```python
from build123d import *

# Parameters (mm, degrees)
STOCK_DGT_START                               = 10.16
STOCK_DGT_INSIDE_SWERVE_STRUCTURE_SM_2_R      = 1.905
STOCK_DGT_INSIDE_SWERVE_STRUCTURE_SM_2_R_2    = 1.5
STOCK_DGT_INSIDE_SWERVE_STRUCTURE_SM_2_R_3    = 4.7625
STOCK_DGT_INSIDE_SWERVE_STRUCTURE_SMALL_DEPTH = 2.286
CUT_EXTRUDE2_DEPTH                            = 66.309248357
FILLET1_R                                     = 2.54
FILLET2_R                                     = 1.27
CHAMFER1_SIZE                                 = 1.27


# Read off the part's stored shape, not the designer's step: Stock-DGT inside swerve structure Small Bearing-1
with BuildPart() as part:
    # Stock-DGT inside swerve structure Sm 2 → Stock-DGT inside swerve structure Small Bearing-1 (new body)
    with BuildSketch(Plane.YZ.offset(STOCK_DGT_START)):
        with BuildLine():
            ThreePointArc((34.33064, -8.13506567), (36.425690436, -10.904598407), (39.07282, -13.152320138))
            Line((39.07282, -13.152320138), (39.07282, -21.59))
            Line((39.07282, -21.59), (56.85282, -21.59))
            Line((56.85282, -21.59), (56.85282, -13.152320138))
            ThreePointArc((56.85282, -13.152320138), (59.499949564, -10.904598407), (61.595, -8.13506567))
            Line((61.595, -8.13506567), (61.595, 8.13506567))
            ThreePointArc((61.595, 8.13506567), (59.499949564, 10.904598407), (56.85282, 13.152320138))
            Line((56.85282, 13.152320138), (56.85282, 21.59))
            Line((56.85282, 21.59), (39.07282, 21.59))
            Line((39.07282, 21.59), (39.07282, 13.152320138))
            ThreePointArc((39.07282, 13.152320138), (36.425690436, 10.904598407), (34.33064, 8.13506567))
            Line((34.33064, 8.13506567), (34.33064, -8.13506567))
        make_face()
        with Locations((42.56532, -18.288)):
            Circle(STOCK_DGT_INSIDE_SWERVE_STRUCTURE_SM_2_R, mode=Mode.SUBTRACT)
        with Locations((41.245305579, -6.717514421)):
            Circle(STOCK_DGT_INSIDE_SWERVE_STRUCTURE_SM_2_R_2, mode=Mode.SUBTRACT)
        with Locations((53.36032, -18.288)):
            Circle(STOCK_DGT_INSIDE_SWERVE_STRUCTURE_SM_2_R, mode=Mode.SUBTRACT)
        with Locations((53.619674249, -5.656854249)):
            Circle(STOCK_DGT_INSIDE_SWERVE_STRUCTURE_SM_2_R_2, mode=Mode.SUBTRACT)
        with Locations((42.305965751, 5.656854249)):
            Circle(STOCK_DGT_INSIDE_SWERVE_STRUCTURE_SM_2_R_2, mode=Mode.SUBTRACT)
        with Locations((42.56532, 18.288)):
            Circle(STOCK_DGT_INSIDE_SWERVE_STRUCTURE_SM_2_R, mode=Mode.SUBTRACT)
        with Locations((47.96282, 0)):
            Circle(STOCK_DGT_INSIDE_SWERVE_STRUCTURE_SM_2_R_3, mode=Mode.SUBTRACT)
        with Locations((54.680334421, 6.717514421)):
            Circle(STOCK_DGT_INSIDE_SWERVE_STRUCTURE_SM_2_R_2, mode=Mode.SUBTRACT)
        with Locations((53.36032, 18.288)):
            Circle(STOCK_DGT_INSIDE_SWERVE_STRUCTURE_SM_2_R, mode=Mode.SUBTRACT)
    extrude(amount=STOCK_DGT_INSIDE_SWERVE_STRUCTURE_SMALL_DEPTH)

    # Sketch2 → Cut-Extrude2 (cut, through all)
    with BuildSketch(Plane.ZY.offset(-10.16)):
        with BuildLine():
            Line((-12.844591897, 56.85282), (-13.152320138, 56.85282))
            ThreePointArc((-13.152320138, 56.85282), (0, 63.83782), (13.152320138, 56.85282))
            Line((13.152320138, 56.85282), (12.844591897, 56.85282))
            ThreePointArc((12.844591897, 56.85282), (0, 63.58382), (-12.844591897, 56.85282))
        make_face()
        with BuildLine():
            Line((13.152320138, 39.07282), (12.844591897, 39.07282))
            ThreePointArc((12.844591897, 39.07282), (0, 32.34182), (-12.844591897, 39.07282))
            Line((-12.844591897, 39.07282), (-13.152320138, 39.07282))
            ThreePointArc((-13.152320138, 39.07282), (0, 32.08782), (13.152320138, 39.07282))
        make_face()
    extrude(amount=-CUT_EXTRUDE2_DEPTH, mode=Mode.SUBTRACT)

    # Fillet1
    fillet1_edges = [part.edges().sort_by_distance(p)[0] for p in [
        (11.303, 34.33064, 7.627536263),
        (11.303, 34.33064, -7.627536263),
        (11.303, 61.595, -7.627536263),
        (11.303, 61.595, 7.627536263),
        (11.303, 56.85282, 12.844591897),
        (11.303, 56.85282, -12.844591897),
        (11.303, 39.07282, -12.844591897),
        (11.303, 39.07282, 12.844591897),
    ]]
    fillet(fillet1_edges, radius=FILLET1_R)

    # Fillet2
    fillet2_edges = [part.edges().sort_by_distance(p)[0] for p in [
        (11.303, 39.07282, 21.59),
        (11.303, 56.85282, 21.59),
        (11.303, 56.85282, -21.59),
        (11.303, 39.07282, -21.59),
    ]]
    fillet(fillet2_edges, radius=FILLET2_R)

    # Chamfer1
    chamfer1_edges = [part.edges().sort_by_distance(p)[0] for p in [
        (12.446, 51.45532, 18.288),
        (12.446, 40.66032, -18.288),
        (12.446, 51.45532, -18.288),
        (12.446, 40.66032, 18.288),
    ]]
    chamfer(chamfer1_edges, length=CHAMFER1_SIZE)


solid = part.part
```
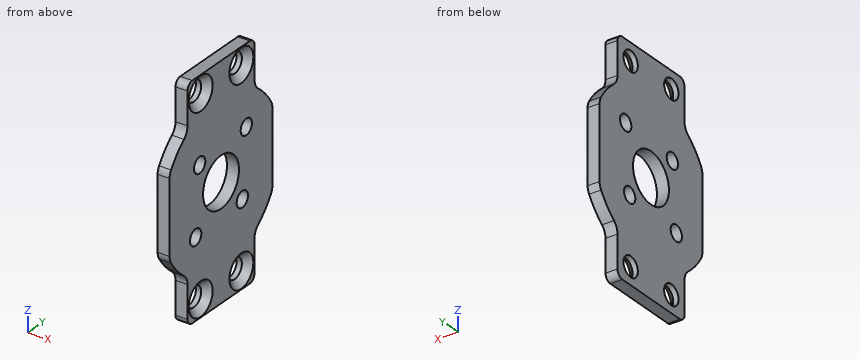
CAD build for the part. Positions are in the model's coordinates, mm. Round coordinates to 2 decimals unless told otherwise and drop trailing zeros. Order: outer loops, then holes, each group sorted by start corner. A loop starts at its lowest first (then second) coordinate and runs counter-clockwise, first axis right, second up.
Item 1: Saw through at B-B on x = 10.65. State how many separate pieces and enclosed holes the cut face has, then the cut area to 3 significant figures.
Item 2: Saw through at A-A on z = 0. Write the cut outline in (x, y) (3 decimals), then the cut area to 3 significant figures.
Item 3: Probe line 1 along Z through (x, y) = (11.75, 55.5); line 2 along Y through (x, z) = (11.9, -6) (3 decimals); line 3 along Y through (x, z) = (11.45, -15.5). List the from-to ranges inside material, lowest first.
Item 4: Pin check, flat tips, straight feed: pin 1 (1.8 mm diameter, centred on y = 53.62, z = -5.66, fed in from -X); pin 2 (1.1 mm diameter, centred on x = 11, z = 17.5, fed in from -Y); pin 3 (6 mm diameter, centred on y = 53.36, z = -18.29, fed in from +X); pin 4 (1.1 mm diameter, centred on x = 11, z = 16.5, fed in from +Y). Stop position of each tip, or through.
Reported:
1. separate pieces: 1
1. enclosed holes: 9
1. area: 824 mm2
2. outline: (10.16, 34.331) - (12.446, 34.331) - (12.446, 43.2) - (10.16, 43.2) - close; (10.16, 52.725) - (12.446, 52.725) - (12.446, 61.595) - (10.16, 61.595) - close
2. area: 40.6 mm2
3. line 1: z = -21.59 to -19.54, -17.04 to 5.46, 7.97 to 17.04, 19.54 to 21.59
3. line 2: y = 34.331 to 39.928, 42.563 to 52.159, 55.08 to 61.595
3. line 3: y = 39.07 to 56.85
4. pin 1: passes through
4. pin 2: stops at y = 39.07
4. pin 3: stops at x = 12.27
4. pin 4: stops at y = 56.85
